Check sheet for the modelled part. Datum: model origin and axes. Units: mm. Give positions to 0.01 mm unless a question says otherwise; leave off trailing zeros. Order: outer loops, then holes, each group sorted by start corner. A loop starts at its lowest first (then second) coordinate and runs counter-clockwise, first axis right, second up.
Item 1: Material ranges on line 1 along X through (y, z) = (-75, 33); line 2 along X through (y, z) = (-99.5, 47); line 3 along Y through (x, z) = (-161, 77.5), recorded low to high.
Item 2: Gauge pin test, flat ends, axial feed: P1, Ø1, axis at x = -68, z = 62, coming from the -Y side; P2, Ø12, axis at x = -12, z = 53.5, coming from the -Y side; P3, Ø4, axis at y = -83, z = 116, coming from the -X side. Record the tip position at first contact, or that the pin passes through.
Item 3: Sectioned sample at A-A on z = 119.5. Record the boundary of the cut face in (x, y), and give its area (3 significant figures).
Item 4: Release check for a two-part mould opening along X. For faces 1 (the cylindrical face through (-125.33, -115.908, 78.264)), 2 (the cylindrical face through (-124.374, -115.024, 78.264)) record: released by +X, released by -X, zero draft, split by the parting line, or undercut.
from build123d import *

# Parameters (mm, degrees)
SKETCH1_R           = 165.062282849
BOSS_EXTRUDE1_DEPTH = 158.75
SHELL1_T            = -1.27
SKETCH2_W           = 163.144728945
SKETCH2_H           = 394.61311295
CUT_EXTRUDE2_DEPTH  = 158.75
SKETCH3_W           = 362.622399732
SKETCH3_H           = 160.71006498
CUT_EXTRUDE3_DEPTH  = 158.75


with BuildPart() as part:
    # Sketch1 → Boss-Extrude1 (new body)
    with BuildSketch(Plane.XY):
        with Locations(Location((-31.532687059, 19.91445928, 0), (0, 0, 180))):
            Circle(SKETCH1_R)
    extrude(amount=BOSS_EXTRUDE1_DEPTH)

    # Shell1
    shell1_openings = [part.faces().sort_by_distance(p)[0] for p in [
        (-31.532687059, 19.91445928, 158.75),
        (-31.532687059, 19.91445928, 0),
    ]]
    offset(amount=SHELL1_T, openings=shell1_openings, kind=Kind.INTERSECTION)

    # Sketch2 → Cut-Extrude2 (cut)
    with BuildSketch(Plane.XY.offset(158.75)):
        with Locations((136.971926827, 42.916431228)):
            Rectangle(SKETCH2_W, SKETCH2_H)
    extrude(amount=-CUT_EXTRUDE2_DEPTH, mode=Mode.SUBTRACT)

    # Sketch3 → Cut-Extrude3 (cut)
    with BuildSketch(Plane.XY.offset(158.75)):
        with Locations((-34.997933009, 126.669881209)):
            Rectangle(SKETCH3_W, SKETCH3_H)
    extrude(amount=-CUT_EXTRUDE3_DEPTH, mode=Mode.SUBTRACT)


solid = part.part
Report:
1. line 1: x = -166.58 to -165.02
1. line 2: x = -145.49 to -143.64
1. line 3: y = -82.48 to -80.42
2. P1: stops at y = -141.18
2. P2: stops at y = -144.59
2. P3: stops at x = -162.15
3. outline: (-194.47, 46.31) arc R165.06 ccw to (55.4, -120.4) - (55.4, -118.9) arc R163.79 cw to (-193.18, 46.31) - close
3. area: 478 mm2
4. face 1: split by the parting line
4. face 2: undercut
